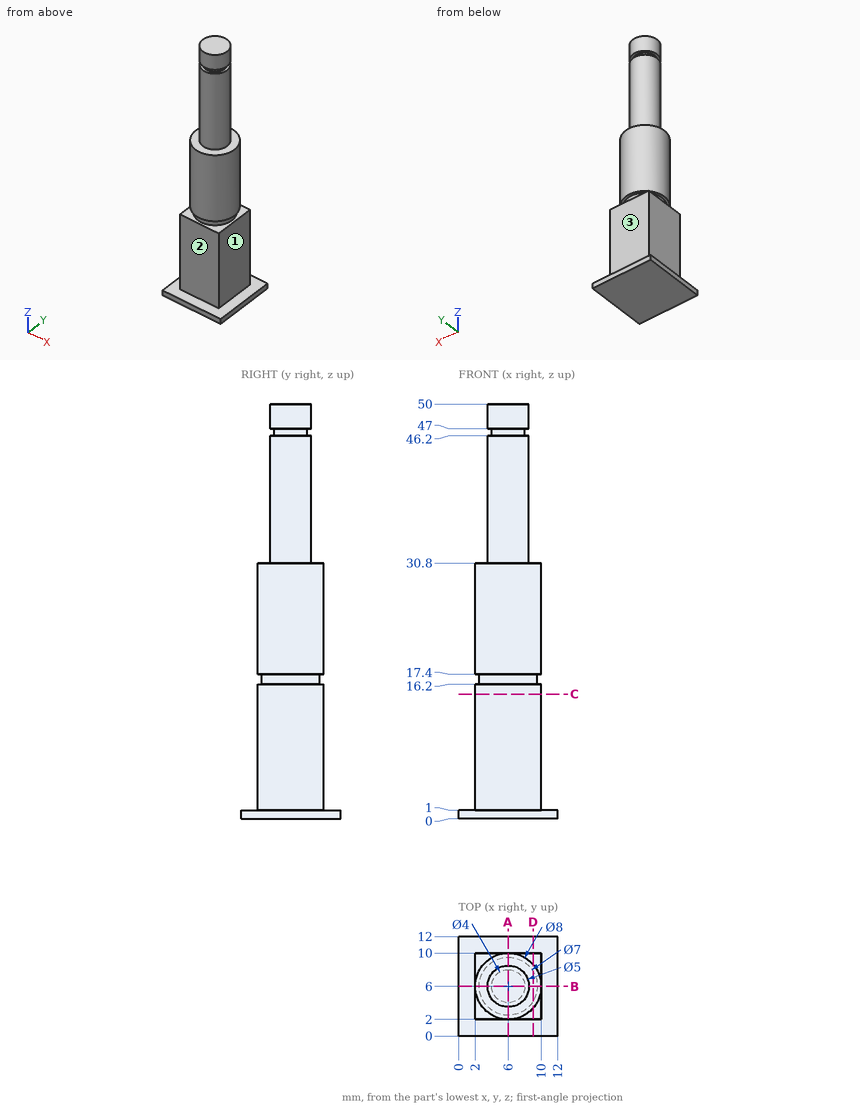
Source: three-view drawing plus pictorial views. Frame: mm from the lowest corner of the part. A direction names the side the tool comes from. Round coordinates to 2 decimals unless told otherwise and drop trailing zeros. Write each loop counter-clockwise with the first axis right and the second up, starting at its lowest first coordinate (ties: lowest second). Pieces come first, ordered by that corner, then holes. Notation, with made-up numbers: M 45.5,36 L 68.5,36 A20 ccw 68.5,75 Z; hole C 65.5,31.25 d3. An arc over 180 degrees is marked long. One line per item, written item: value. Start each with the question number.
Item 1: Section query C-C (z = 15). Return the cut outline in (x, y), plus the area to 3 significant figures.
Item 2: Section query A-A (x = 6). Return the cut outline in (y, z), plus the area to 3 significant figures.
Item 3: Section query D-D (x = 9). Return the cut outline in (y, z), plus the area to 3 significant figures.
Item 4: Set-up query: the marked faces 1, 2 and 3. Return all of +Z, -Z, +X, -X, +Y, -Y with unobstructed straight access to the full face (end or side cutting, diameter ignored); none if empty.
Item 5: Pin query (flat end, axial travel): pin 1 (6.5 mm diameter, centred on y = 4.5, z = 10, fed in from +X); pin 2 (4 mm diameter, centred on y = 9.5, z = 37, fed in from +X); pin 3 (5 mm diameter, centred on y = 10, z = 22.5, fed in from -X); pin 4 (5 mm diameter, centred on x = 6.5, y = 7, fed in from -Z). Return the tip coordinate at first contact, or that it passes through.
Item 6: Ray query, L1, parallel to Z at x = 9, y = 4; L2, parallel to Z at x = 8.5, y = 11; L3, parallel to Z at x = 3.75, y = 6. Return the intervals inside material, ascending. Write a range as from..to.
Result set:
1. outline: M 2,2 L 10,2 L 10,10 L 2,10 Z
1. area: 64.0 mm²
2. outline: M 0,0 L 12,0 L 12,1 L 10,1 L 10,16.2 L 9.5,16.2 L 9.5,17.4 L 10,17.4 L 10,30.8 L 8.5,30.8 L 8.5,46.2 L 8,46.2 L 8,47 L 8.5,47 L 8.5,50 L 3.5,50 L 3.5,47 L 4,47 L 4,46.2 L 3.5,46.2 L 3.5,30.8 L 2,30.8 L 2,17.4 L 2.5,17.4 L 2.5,16.2 L 2,16.2 L 2,1 L 0,1 Z
2. area: 344 mm²
3. outline: M 0,0 L 12,0 L 12,1 L 10,1 L 10,16.2 L 7.8,16.2 L 7.8,17.4 L 8.65,17.4 L 8.65,30.8 L 3.35,30.8 L 3.35,17.4 L 4.2,17.4 L 4.2,16.2 L 2,16.2 L 2,1 L 0,1 Z
3. area: 209 mm²
4. face 1: +Z, +X, +Y, -Y
4. face 2: +Z, +X, -X, -Y
4. face 3: +Z, +X, -X, +Y
5. pin 1: stops at x = 10
5. pin 2: stops at x = 8
5. pin 3: stops at x = 2.29
5. pin 4: stops at z = 0
6. L1: z = 0..16.2, 17.4..30.8
6. L2: z = 0..1
6. L3: z = 0..46.2, 47..50
